Check sheet for the drawn part. Datum: minimum x, y, z corner. Units: mm. A direction names the side the tool comes from. Give positions to 0.01 mm unless a question says otherwise; leave off trailing zeros. Write each loop counter-clockwise with the first axis right and the second up, starting at its lowest first coordinate (ties: lowest second). Pieces come first, ordered by that corner, then holes. Notation, with made-up numbers: M -13,72.5 L 29,72.5 A9 ccw 29,83.5 Z; hole C 76.5,74 d11. An arc over 180 degrees is marked long. Write item = value, one per line. Start each with the question number.
1) Sectioned sample at B-B, the plane x = 5. Record the cut outline in (y, z).
2) Set-up check for the marked faces 1 and 2: record each of +Z, -Z, +X, -X, +Y, -Y from which the full face is reachable in a straight line by a thin tool's end or side.
3) Sectioned sample at C-C, the plane z = 43. Record the cut outline in (x, y).
4) Gauge pin test, flat ends, axial feed: pin 1 (1 mm diameter, centred on x = 8, z = 106, fed in from -Y); pin 2 (6 mm diameter, centred on x = 9, z = 15, fed in from +Y); pin 3 (6 mm diameter, centred on x = 12.5, z = 34.5, fed in from +Y). Record the tip position at first contact, or that the pin passes through.
5) Sectioned sample at A-A, the plane y = 7.5. Record the cut outline in (x, z).
6) Sectioned sample at D-D, the plane x = 13.5. Record the cut outline in (y, z).
7) Scan lines: L1, parallel to Z at x = 12.5, y = 9.75; L2, parallel to X at y = 7.5, z = 91.5; L3, parallel to X at y = 8.5, z = 108. Record each from-to range of solid material in increasing order.
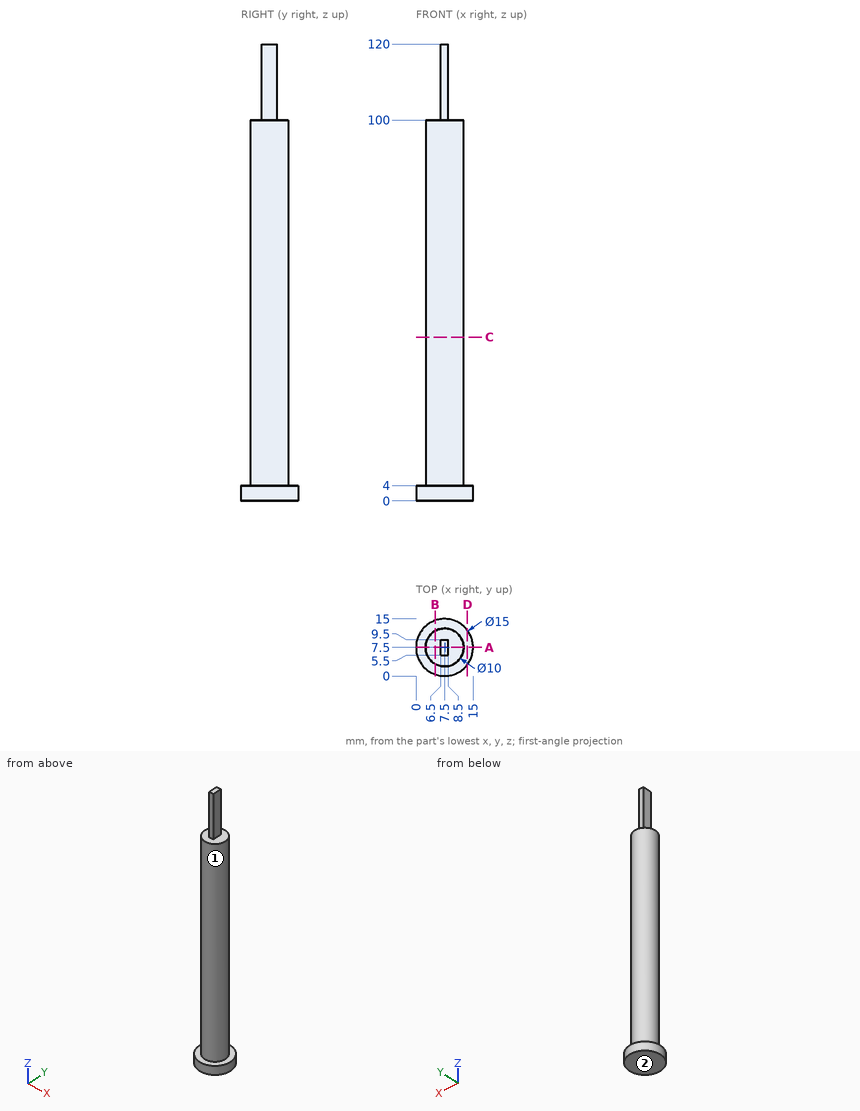
Data:
q1.outline = M 0.43,0 L 14.57,0 L 14.57,4 L 11.83,4 L 11.83,100 L 3.17,100 L 3.17,4 L 0.43,4 Z
q2.face_1 = +Z
q2.face_2 = -Z, +X, -X, +Y, -Y
q3.outline = C 7.5,7.5 d10
q4.pin_1 = 5.5
q4.pin_2 = 12.5
q4.pin_3 = 12.08
q5.outline = M 0,0 L 15,0 L 15,4 L 12.5,4 L 12.5,100 L 8.5,100 L 8.5,120 L 6.5,120 L 6.5,100 L 2.5,100 L 2.5,4 L 0,4 Z
q6.outline = M 3,0 L 12,0 L 12,4 L 3,4 Z
q7.L1 = 0 to 4
q7.L2 = 2.5 to 12.5
q7.L3 = 6.5 to 8.5
